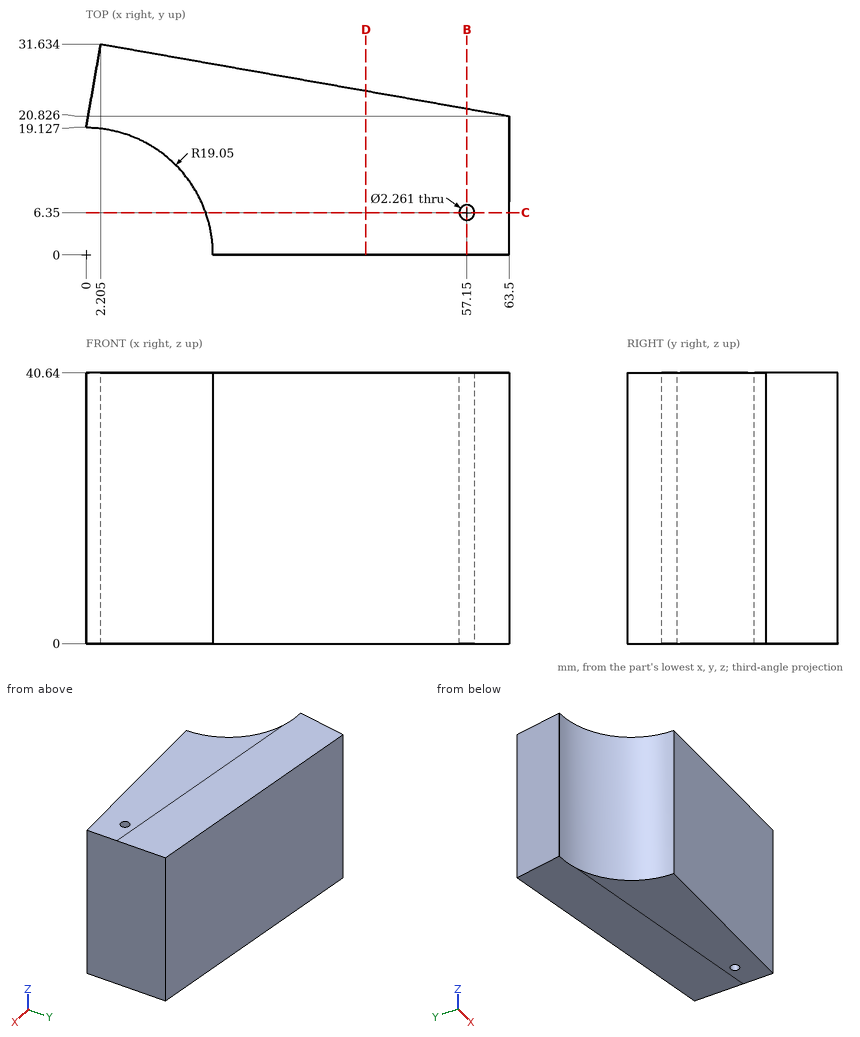
Geometry check sheet. Reference: drawing and pictorial views, mm from the part's lowest x, y, z. Round coordinates to 2 decimals unless told otherwise and drop trailing zeros. Write each loop counter-clockwise with the first axis right and the second up, starting at its lowest first coordinate (ties: lowest second). Pieces come first, ordered by that corner, then holes. Notation, with made-up numbers: (-33.5, 36.5) -> (5.5, 36.5) arc R21 ccw to (5.5, 70.5) -> close; hole circle Ø3 at (79, 30.25). An arc over 180 degrees is marked (long way). One line per question, with ' | ' between items. Start each with the question number.
1. Sectioned sample at D-D, the plane x = 42. Record the cut outline in (y, z), then the cut area to 3 significant figures.
2. Sectioned sample at B-B, the plane x = 57.15. Record the cut outline in (y, z), then the cut area to 3 significant figures.
3. Sectioned sample at C-C, the plane y = 6.35. Record the cut outline in (x, z).
4. Depth check by flat-ended pin: pin 1 (1.4 mm diameter, centred on x = 57.15, y = 6.35, fed in from -Z) (1 decimal); pin 2 (5 mm diameter, centred on y = 26.5, z = 17, fed in from -X); pin 3 (3 mm diameter, centred on x = 8, z = 9.5, fed in from +Y); pin 4 (1 mm diameter, centred on x = 24.5, z = 17, fed in from +Y). Enter the tip coordinate at first touch or a pass-through.
5. Scan lines: line 1 along Y through (x, z) = (57.15, 26) (1 decimal); line 2 along X through (y, z) = (6, 14) (1 decimal); line 3 along X through (y, z) = (10, 6.5) (1 decimal). Record each from-to range of solid material in increasing order. Write a range as from..to.
Taken from the geometry:
1) outline: (0, 0) -> (24.62, 0) -> (24.62, 40.64) -> (0, 40.64) -> close | area: 1,000 mm^2
2) outline: (0, 0) -> (5.22, 0) -> (5.22, 40.64) -> (0, 40.64) -> close; (7.48, 0) -> (21.95, 0) -> (21.95, 40.64) -> (7.48, 40.64) -> close | area: 800 mm^2
3) outline: (17.96, 0) -> (56.02, 0) -> (56.02, 40.64) -> (17.96, 40.64) -> close; (58.28, 0) -> (63.5, 0) -> (63.5, 40.64) -> (58.28, 40.64) -> close
4) pin 1: passes through | pin 2: stops at x = 0.86 | pin 3: stops at y = 30.88 | pin 4: stops at y = 27.79
5) line 1: y = 0..5.2, 7.5..21.9 | line 2: x = 18.1..56.1, 58.2..63.5 | line 3: x = 16.2..63.5
